Check sheet for the modelled part. Datum: model origin and axes. Units: mm. A direction names the side the tool comes from. Round coordinates to 2 decimals unless told otherwise and drop trailing zeros. Order: outer loops, then holes, each group sorted by start corner. A loop starts at its lowest first (then second) coordinate and runs counter-clockwise, first axis right, second up. Notation, with made-up numbers: (-1.75, 2.25) -> (44.25, 2.25) arc R28 cw to (44.25, 39.25) -> close; hole circle Ø11 at (55.25, -20.5). An arc over 180 degrees is marked (long way). Use CSV: the item, a comma, the result in double quotes.
```python
from build123d import *

# Parameters (mm, degrees)
CUT_EXTRUDE2_DEPTH = 1.155


with BuildPart() as part:
    # Sketch10 → Revolve3 (revolve)
    with BuildSketch(Plane(origin=(0, 0, 0), x_dir=(0, 0, -1), z_dir=(1, 0, 0)), mode=Mode.PRIVATE) as revolve3_sk:
        Polygon((13.275, 1.5), (13.65, 1.125), (13.65, 0), (1.65, 0), (1.65, 1.5), align=None)
    revolve(revolve3_sk.sketch.rotate(Axis((0, 0, 0), (0, 0, -1)), 90), axis=Axis((0, 0, 0), (0, 0, -1)))

    # Sketch7 → Revolve2 (revolve)
    with BuildSketch(Plane(origin=(0, 0, 0), x_dir=(0, 0, -1), z_dir=(1, 0, 0)), mode=Mode.PRIVATE) as revolve2_sk:
        with BuildLine():
            Line((1.4025, 2.85), (1.65, 2.85))
            Line((1.65, 2.85), (1.65, 0))
            Line((1.65, 0), (0, 0))
            Line((0, 0), (0, 1.5))
            ThreePointArc((0, 1.5), (0.59512511, 2.285251969), (1.4025, 2.85))
        make_face()
    revolve(revolve2_sk.sketch.rotate(Axis((0, 0, 0), (0, 0, -1)), 180), axis=Axis((0, 0, 0), (0, 0, -1)))

    # Sketch5 → Cut-Extrude2 (cut)
    with BuildSketch(Plane.XY):
        Polygon((1, -0.577350269), (1, 0.577350269), (0, 1.154700538), (-1, 0.577350269), (-1, -0.577350269), (0, -1.154700538), align=None)
    extrude(amount=-CUT_EXTRUDE2_DEPTH, mode=Mode.SUBTRACT)

    # Cut-Extrude3 cone 1 section (through the dimple's axis) → Cut-Extrude3 (revolve, cut)
    with BuildSketch(Plane(origin=(0, 0, 0), x_dir=(0, -1, 0), z_dir=(1, 0, 0))):
        Polygon((0, 0), (1.154700538, 0), (0, 1.154700538), align=None)
    revolve(axis=Axis((0, 0, 0), (0, 0, -1)), mode=Mode.SUBTRACT)


with BuildPart() as body_2:
    # Split1: read off the stored shape, not the designer's step
    # Split1: the piece on the far side of the plane
    add(part.part)
    split(bisect_by=Plane.XY.offset(-1.65), keep=Keep.BOTTOM)


with BuildPart() as part_1:
    add(part.part)

    # Split1
    split(bisect_by=Plane.XY.offset(-1.65), keep=Keep.TOP)


with BuildPart() as body_2_1:
    add(body_2.part)

    # Boss-Extrude1: read off the stored shape, not the designer's step
    # Boss-Extrude1: union part
    add(part_1.part)


solid = body_2_1.part
```
Q1. Mould release check, pull along X, two halves, no side actions. Record for faces 3 (the face through (0, 0, -13.65)), 4 (the face through (0.49, -0.87, -0.57)), 5 (the face through (1.43, -0.45, -7.54)): pulls with the +X half, pulls with the -X half, needs draft (parallel to the pull), parting line crosses it, or undercut.
Result sheet:
face 3,"needs draft"
face 4,"undercut"
face 5,"parting line crosses it"
Q2. Sectioned sample at D-D, the plane y = -2.15. Enter the section's corners in (x, z), then the cut area to 3 significant figures.
Result sheet:
outline,"(-1.87, -1.65) -> (1.87, -1.65) -> (1.87, -1.4) arc R2.33 ccw to (-1.87, -1.4) -> close"
area,"3.38 mm^2"
Q3. Sectioned sample at B-B, the plane z = -10. Enter the section's corners in (x, y), then the cut area to 3 significant figures.
Result sheet:
outline,"circle Ø3 at (0, 0)"
area,"7.07 mm^2"
Q4. Go/stop test with a flat-tipped pin: pin 1 (3 mm diameter, centred on y = 1.5, z = -5, fed in from +X). Record where the tip stops, or that it passes through.
Result sheet:
pin 1,"stops at x = 1.5"
Q5. Sectioned sample at C-C, the plane x = -2.25. Enter the section's corners in (y, z).
Result sheet:
outline,"(-1.75, -1.65) -> (1.75, -1.65) -> (1.75, -1.4) arc R2.24 ccw to (-1.75, -1.4) -> close"
Q6. Scan lines: L1, parallel to Z at x = 0.55, y = 0.8 (3 decimals); L2, parallel to X at y = 0.4, z = -10.5; L3, parallel to Y at x = -0.85, z = -2.5. Record each from-to range of solid material in increasing order.
Result sheet:
L1,"z = -13.65 to -1.155"
L2,"x = -1.45 to 1.45"
L3,"y = -1.24 to 1.24"
Q7. Access from +Z, -Z, +X, -X, +Y, -Y to the whole of each face (thin tool, end or side, straight path). Record for faces 1 (the face through (-0.51, -0.86, -0.57)), 2 (the face through (1.2, -1.2, -1.65)).
Result sheet:
face 1,"+Z"
face 2,"-Z"
